Input: dimensioned drawing with shaded views. Units: mm. Origin: part minimum x, y, z. A direction names the side the tool comes from. Round coordinates to 2 decimals unless told otherwise and drop trailing zeros. Loops run counter-clockwise (first coordinate to the right, second up) from the corner with the lowest first, then second, coordinate; pieces in that order, holes last. Notation, with made-up numbers: (35, -11.5) - (94, -11.5) arc R32 ccw to (94, 27.5) - close; hole circle Ø5 at (75.5, -6.75). An arc over 180 degrees is marked (long way). Answer as a JSON object with one key per item and string values. Group by question number.
Item 1: Draft query along X for the marked faces 1, 2 and 3. Return one class per face: released by +X, released by -X, zero draft, split by the parting line, or undercut.
Item 2: Section D-D (z = 11). Return the cut outline in (x, y).
Item 3: First-contact query: pin 1 (4 mm diameter, centred on x = 23.5, y = 4, fed in from +Z); pin 2 (6 mm diameter, centred on y = 5.5, z = 10, fed in from -X); pin 3 (3 mm diameter, centred on y = 3, z = 7.5, fed in from +X). Flat tips, straight axial feed; report the tip coordinate or a pass-through.
Item 4: Reachability of the marked faces 4 and 5 from +Z, -Z, +X, -X, +Y, -Y: full face, straight path, thin tool, end or side. Return the list, or none.
Item 5: Line query: line 1 (X direction, y = 5, z = 0.35); line 2 (X direction, y = 8.5, z = 8.25); line 3 (Y direction, x = 45, z = 0.5). Output: solid intervals per line, ascending.
Item 6: Section B-B (z = 4). Return the cut outline in (x, y), plus the area to 3 significant figures.
Item 7: Section A-A (x = 5). Return the cut outline in (y, z), plus the area to 3 significant figures.
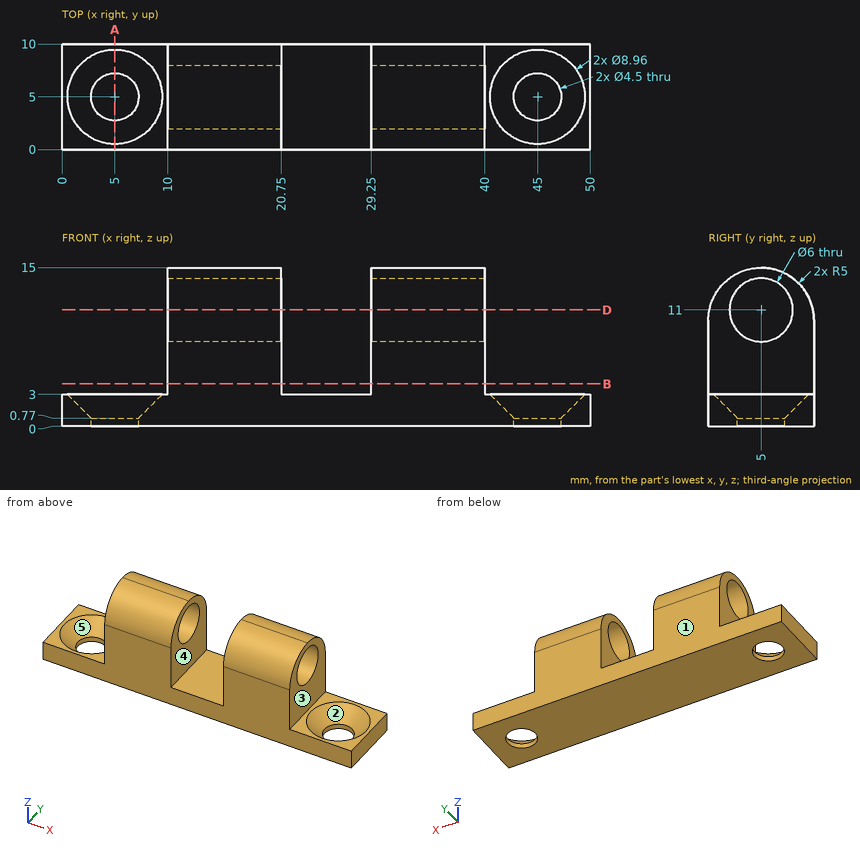
Values:
{
 "1": {"face 1": "zero draft", "face 2": "undercut", "face 3": "released by +X"},
 "2": {"outline": "(10, 0.1) - (20.75, 0.1) - (20.75, 2) - (10, 2) - close; (10, 8) - (20.75, 8) - (20.75, 9.9) - (10, 9.9) - close; (29.25, 0.1) - (40, 0.1) - (40, 2) - (29.25, 2) - close; (29.25, 8) - (40, 8) - (40, 9.9) - (29.25, 9.9) - close"},
 "3": {"pin 1": "stops at z = 3", "pin 2": "stops at x = 10", "pin 3": "stops at x = 40"},
 "4": {"face 4": "+Z, +Y, -Y", "face 5": "+Z"},
 "5": {"line 1": "x = 0 to 2.75, 7.25 to 42.75, 47.25 to 50", "line 2": "x = 10 to 20.75, 29.25 to 40", "line 3": "y = 0 to 2.75, 7.25 to 10"},
 "6": {"outline": "(10, 0) - (20.75, 0) - (20.75, 10) - (10, 10) - close; (29.25, 0) - (40, 0) - (40, 10) - (29.25, 10) - close", "area": "215 mm^2"},
 "7": {"outline": "(0, 0) - (2.75, 0) - (2.75, 0.77) - (0.52, 3) - (0, 3) - close; (7.25, 0) - (10, 0) - (10, 3) - (9.48, 3) - (7.25, 0.77) - close", "area": "11.5 mm^2"}
}
